from build123d import *

# Parameters (mm, degrees)
SKETCH1_W               = 120
SKETCH1_H               = 15
BOSS_EXTRUDE1_DEPTH     = 1
FILLET1_R               = 3
SKETCH3_R               = 1.25
CUT_EXTRUDE1_DEPTH      = 1
MIRROR2_COPY_1_SKETCH_R = 1.25
MIRROR2_COPY_1_DEPTH    = 1


with BuildPart() as part:
    # Sketch1 → Boss-Extrude1 (new body)
    with BuildSketch(Plane(origin=(0, 0, 0), x_dir=(1, 0, 0), z_dir=(0, 1, 0))):
        Rectangle(SKETCH1_W, SKETCH1_H)
    extrude(amount=BOSS_EXTRUDE1_DEPTH)

    # Fillet1
    fillet1_edges = [part.edges().sort_by_distance(p)[0] for p in [
        (60, 0.5, 7.5),
        (-60, 0.5, 7.5),
        (-60, 0.5, -7.5),
        (60, 0.5, -7.5),
    ]]
    fillet(fillet1_edges, radius=FILLET1_R)

    # Sketch3 → Cut-Extrude1 (cut)
    with BuildSketch(Plane(origin=(0, 1, 0), x_dir=(1, 0, 0), z_dir=(0, 1, 0))):
        with Locations((-57.5, 5)):
            Circle(SKETCH3_R)
    cut_extrude1 = extrude(amount=-CUT_EXTRUDE1_DEPTH, mode=Mode.SUBTRACT)

    # Mirror1: Cut-Extrude1 across plane
    add(cut_extrude1.mirror(Plane.XY), mode=Mode.SUBTRACT)

    # Mirror2: Cut-Extrude1 across plane
    add(cut_extrude1.mirror(Plane(origin=(0, 0, 0), x_dir=(0, 0, 1), z_dir=(1, 0, 0))), mode=Mode.SUBTRACT)

    # Mirror2 copy 1 sketch → Mirror2 copy 1 (cut)
    with BuildSketch(Plane(origin=(0, 1, 0), x_dir=(-1, 0, 0), z_dir=(0, 1, 0))):
        with Locations((-57.5, 5)):
            Circle(MIRROR2_COPY_1_SKETCH_R)
    extrude(amount=-MIRROR2_COPY_1_DEPTH, mode=Mode.SUBTRACT)


solid = part.part
Can you work these out from the model? Positions are in its coordinate system, mm. Coordinates: 2 decimals unless noted, no trailing zeros. Loops run counter-clockwise (first coordinate to the right, second up) from the corner with the lowest first, then second, coordinate; pieces in that order, holes last. Notation, with made-up numbers: (43, 54.25) - (74, 54.25) arc R32 cw to (74, 82.25) - close; hole circle Ø10 at (26, -31). An arc over 180 degrees is marked (long way). Put each result on its own line as item: value. Start each with the question number.
Item 1: If I drill on line 1 along X through (y, z) = (0.5, -6); line 2 along X through (y, z) = (0.4, -5); line 3 along Z through (x, y) = (-57.5, 0.6), over which ranges is the centre line in solid material (lowest first)?
Item 2: For pin 1 (2 mm diameter, centred on x = 57.5, z = -5, fed in from +Y) (3 decimals), with a flat end and sliding along its axis, tell me the tip position at first contact or that it passes through.
Item 3: Suppose I cut it at A-A (y = 0.45). Please give me the cut outline in (x, z), and give its area (3 significant figures).
Item 4: If we mould it in two halves opening along X, with no side actions, what happens to faces 1 (the face through (-1, 0, 0)), 2 (the face through (-56.31, 0.51, 5.38)), 3 (the face through (-59.14, 0.51, 6.6)), 4 (the face through (56.31, 0.51, -5.38))? For each: +X half, -X half, draft (parallel to the pull), parting line (faces both ways), or undercut.
Here are the results:
1. line 1: -59.6 to -58.25, -56.75 to 56.75, 58.25 to 59.6
1. line 2: -59.96 to -58.75, -56.25 to 56.25, 58.75 to 59.96
1. line 3: -7.46 to -6.25, -3.75 to 3.75, 6.25 to 7.46
2. pin 1: through
3. outline: (-60, -4.5) arc R3 ccw to (-57, -7.5) - (57, -7.5) arc R3 ccw to (60, -4.5) - (60, 4.5) arc R3 ccw to (57, 7.5) - (-57, 7.5) arc R3 ccw to (-60, 4.5) - close; hole circle Ø2.5 at (-57.5, -5); hole circle Ø2.5 at (-57.5, 5); hole circle Ø2.5 at (57.5, -5); hole circle Ø2.5 at (57.5, 5)
3. area: 1,770 mm²
4. face 1: draft
4. face 2: undercut
4. face 3: -X half
4. face 4: undercut
